Geometry: final body of the model. Coordinates: model frame, mm. A direction names the side the tool comes from. Give positions to 0.01 mm unless a question says otherwise; leave off trailing zeros. Write each loop counter-clockwise with the first axis right and the second up, starting at its lowest first coordinate (ties: lowest second). Pieces come first, ordered by that corner, then holes. Notation, with made-up numbers: (-15.5, 47.5) -> (2.5, 47.5) arc R24 cw to (2.5, 81.5) -> close; hole circle Ø3 at (25, 11). An arc over 180 degrees is marked (long way). Use CSV: the item, a comma, the result in double quotes. Start each with the question number.
1) Section C-C (x = 0). Output: boundary loops of the cut face in (y, z), plus the area to 3 significant figures.
2) Section A-A (z = 0). Output: boundary loops of the cut face in (x, y), plus the area to 3 significant figures.
3) Material intervals for line 1 (Y direction, x = 39.5, z = -37); line 2 (Z direction, x = 52.5, y = 82.5); line 3 (Y direction, x = 4, z = 25.5), sorted ascending. Write a range as [from, to].
4) Contact query for a flat-ended pin moving along its axis: P1, Ø3, axis at y = 15, z = -11.5, coming from the +X side. Output: stop coordinate, or through.
5) Section B-B (y = 70). Output: boundary loops of the cut face in (x, z), plus the area to 3 significant figures.
6) Set-up query: faces 1 (the face through (-15.456, 12.522, -20.157)), 2 (the face through (-49.91, 84.18, -49.51)). Return all of +Z, -Z, +X, -X, +Y, -Y with unobstructed straight access to the full face (end or side cutting, diameter ignored); none if empty.
7) Section D-D (x = 27.5). Output: boundary loops of the cut face in (y, z), plus the area to 3 significant figures.
```python
from build123d import *

# Parameters (mm, degrees)
SKETCH1_R           = 25.4
BOSS_EXTRUDE1_DEPTH = 25.4
SKETCH3_W           = 114.3
SKETCH3_H           = 114.3
BOSS_EXTRUDE2_DEPTH = 50.8
FILLET1_R           = 25.4


with BuildPart() as part:
    # Sketch1 → Boss-Extrude1 (new body)
    with BuildSketch(Plane(origin=(0, 0, 0), x_dir=(1, 0, 0), z_dir=(0, 1, 0))):
        with Locations(Location((0, 0, 0), (0, 0, 270))):
            Circle(SKETCH1_R)
    extrude(amount=BOSS_EXTRUDE1_DEPTH)

    # Sketch2 one side → Revolve1 (revolve)
    with BuildSketch(Plane.XY):
        with BuildLine():
            Line((25.4, 25.4), (0, 25.4))
            Line((0, 25.4), (0, 17.427972806))
            ThreePointArc((0, 17.427972806), (13.310834098, 19.467783044), (25.4, 25.4))
        make_face()
        with BuildLine():
            ThreePointArc((44.45, 61.877972806), (31.430896424, 93.308869229), (0, 106.327972806))
            Line((0, 106.327972806), (0, 25.4))
            Line((0, 25.4), (25.4, 25.4))
            ThreePointArc((25.4, 25.4), (39.400713826, 41.301621088), (44.45, 61.877972806))
        make_face()
    revolve(axis=Axis((0, 145.460296173, 0), (0, -1, 0)))

    # Sketch3 → Boss-Extrude2 (add)
    with BuildSketch(Plane(origin=(0, 58.42, 0), x_dir=(1, 0, 0), z_dir=(0, 1, 0))):
        Rectangle(SKETCH3_W, SKETCH3_H)
    extrude(amount=BOSS_EXTRUDE2_DEPTH)

    # Fillet1
    fillet1_edges = [part.edges().sort_by_distance(p)[0] for p in [
        (-57.15, 83.82, 57.15),
        (57.15, 83.82, 57.15),
        (57.15, 83.82, -57.15),
        (-57.15, 83.82, -57.15),
    ]]
    fillet(fillet1_edges, radius=FILLET1_R)


solid = part.part
```
Answers follow:
1,outline,"(0, -25.4) -> (25.4, -25.4) arc R44.45 ccw to (58.42, -44.32) -> (58.42, -57.15) -> (109.22, -57.15) -> (109.22, 57.15) -> (58.42, 57.15) -> (58.42, 44.32) arc R44.45 ccw to (25.4, 25.4) -> (0, 25.4) -> close"
1,area,"9,620 mm^2"
2,outline,"(-57.15, 58.42) -> (-44.32, 58.42) arc R44.45 ccw to (-25.4, 25.4) -> (-25.4, 0) -> (25.4, 0) -> (25.4, 25.4) arc R44.45 ccw to (44.32, 58.42) -> (57.15, 58.42) -> (57.15, 109.22) -> (-57.15, 109.22) -> close"
2,area,"9,620 mm^2"
3,line 1,"y = [58.42, 109.22]"
3,line 2,"z = [-46.4, 46.4]"
3,line 3,"y = [25.69, 109.22]"
4,P1,"stops at x = 23.35"
5,outline,"(-57.15, -31.75) arc R25.4 ccw to (-31.75, -57.15) -> (31.75, -57.15) arc R25.4 ccw to (57.15, -31.75) -> (57.15, 31.75) arc R25.4 ccw to (31.75, 57.15) -> (-31.75, 57.15) arc R25.4 ccw to (-57.15, 31.75) -> close"
5,area,"12,500 mm^2"
6,face 1,"-Y"
6,face 2,"-Z, -X, +Y, -Y"
7,outline,"(58.42, -57.15) -> (109.22, -57.15) -> (109.22, 57.15) -> (58.42, 57.15) -> (58.42, 34.75) arc R34.92 ccw to (58.42, -34.75) -> close"
7,area,"7,480 mm^2"
